Can you work these out from the model? Positions are in its coordinate system, mm. Face numbers are marked on the shaded views. A direction names the side the tool comes from. Give positions to 0.01 mm unless a question says otherwise; leave off trailing zeros. Loops run counter-clockwise (first coordinate to the right, second up) from the corner with the lowest first, then second, coordinate; pieces in that order, holes last. Notation, with made-up numbers: M -7,13.25 L 38,13.25 A32 cw 38,47.25 Z; hole C 73.5,75 d4. An arc over 180 degrees is marked long. Use CSV: the item, a comma, the result in double quotes.
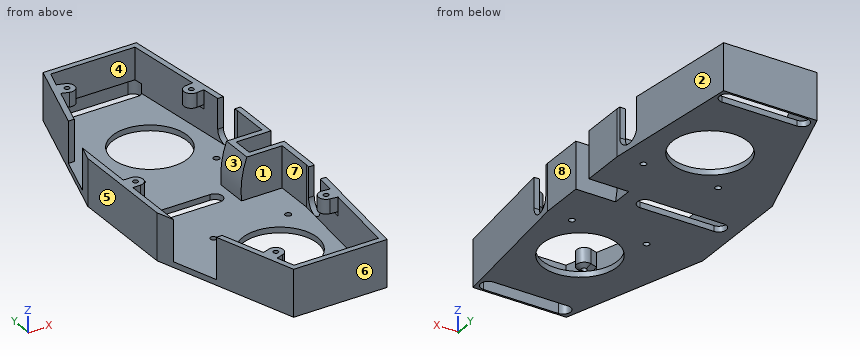
from build123d import *

# Parameters (mm, degrees)
EXTRUDE1_DEPTH          = 40
CHAMFER1_SIZE           = 20
CHAMFER1_SIZE2          = 11.547005384
CUT_EXTRUDE1_DEPTH      = 3
CUT_EXTRUDE1_DEPTH_BACK = 8
SKETCH4_R               = 45
SHELL2_T                = -3
SKETCH6_W               = 125.382075166
SKETCH6_H               = 262.961923039
CUT_EXTRUDE3_DEPTH      = 15
SKETCH7_W               = 55
SKETCH7_H               = 124
CUT_EXTRUDE4_DEPTH      = 22
CUT_EXTRUDE5_DEPTH      = 5
CUT_EXTRUDE5_DEPTH_BACK = 12
SKETCH8_R               = 20
SKETCH8_R_2             = 1.6
CUT_EXTRUDE6_DEPTH      = 10
SKETCH10_R              = 1.35
EXTRUDE2_DEPTH          = 10
CHAMFER2_SIZE           = 2.309401077
CHAMFER2_SIZE_2         = 4


with BuildPart() as part:
    # Sketch2 → Extrude1 (new body)
    with BuildSketch(Plane.XY):
        Polygon((24.967783135, -105), (33.5, -29), (33.5, 29), (24.967783135, 105), (-24.967783135, 105), (-49.5, 29), (-49.5, -29), (-24.967783135, -105), align=None)
    extrude(amount=EXTRUDE1_DEPTH)

    # Chamfer1
    chamfer1_edges = [part.edges().sort_by_distance(p)[0] for p in [
        (0, -105, 40),
        (29.233891568, -67, 40),
        (33.5, 0, 40),
        (29.233891568, 67, 40),
        (0, 105, 40),
        (-37.233891568, 67, 40),
        (-49.5, 0, 40),
        (-37.233891568, -67, 40),
    ]]
    chamfer1_side = [part.faces().sort_by_distance(p)[0] for p in [
        (-5.515477183, 0, 40),
    ]]
    chamfer(chamfer1_edges, length=CHAMFER1_SIZE, length2=CHAMFER1_SIZE2, reference=chamfer1_side[0])

    # Sketch4 → Cut-Extrude1 (cut, two sides: drawn at the far end of the back side and taken through both)
    with BuildSketch(Plane.XZ.offset(2.5).offset(-CUT_EXTRUDE1_DEPTH_BACK)):
        with Locations((56.5, 8)):
            Circle(SKETCH4_R)
    extrude(amount=CUT_EXTRUDE1_DEPTH + CUT_EXTRUDE1_DEPTH_BACK, mode=Mode.SUBTRACT)

    # Shell2
    shell2_openings = [part.faces().sort_by_distance(p)[0] for p in [
        (-6.280046319, 0, 40),
    ]]
    offset(amount=SHELL2_T, openings=shell2_openings, kind=Kind.INTERSECTION)

    # Sketch6 → Cut-Extrude3 (cut)
    with BuildSketch(Plane.XY.offset(40)):
        with Locations((5.510547988, -25.491958467)):
            Rectangle(SKETCH6_W, SKETCH6_H)
    extrude(amount=-CUT_EXTRUDE3_DEPTH, mode=Mode.SUBTRACT)

    # Sketch7 → Cut-Extrude4 (cut)
    with BuildSketch(Plane.XY.offset(25)):
        with Locations((-19, 0)):
            Rectangle(SKETCH7_W, SKETCH7_H)
    extrude(amount=-CUT_EXTRUDE4_DEPTH, mode=Mode.SUBTRACT)

    # Sketch8 → Cut-Extrude5 (cut, two sides: drawn at the far end of the back side and taken through both)
    with BuildSketch(Plane.XY.offset(3).offset(-CUT_EXTRUDE5_DEPTH_BACK)):
        with Locations((0, 54.5)):
            Circle(SKETCH8_R)
        with Locations((0, -54.5)):
            Circle(SKETCH8_R)
        with Locations((19.967783135, -30)):
            Circle(SKETCH8_R_2)
        with Locations((-19.967783135, -30)):
            Circle(SKETCH8_R_2)
        with Locations((19.967783135, 30)):
            Circle(SKETCH8_R_2)
        with Locations((-19.967783135, 30)):
            Circle(SKETCH8_R_2)
        with BuildLine():
            Line((-20.032216865, 104), (19.967783135, 104))
            ThreePointArc((19.967783135, 104), (23.967783135, 100), (19.967783135, 96))
            Line((19.967783135, 96), (-20.032216865, 96))
            ThreePointArc((-20.032216865, 96), (-24.032216865, 100), (-20.032216865, 104))
        make_face()
        with BuildLine():
            Line((-20.032216865, -96), (19.967783135, -96))
            ThreePointArc((19.967783135, -96), (23.967783135, -100), (19.967783135, -104))
            Line((19.967783135, -104), (-20.032216865, -104))
            ThreePointArc((-20.032216865, -104), (-24.032216865, -100), (-20.032216865, -96))
        make_face()
        with BuildLine():
            Line((-39.5, 4), (0, 4))
            ThreePointArc((0, 4), (4, 0), (0, -4))
            Line((0, -4), (-39.5, -4))
            ThreePointArc((-39.5, -4), (-43.5, 0), (-39.5, 4))
        make_face()
    extrude(amount=CUT_EXTRUDE5_DEPTH + CUT_EXTRUDE5_DEPTH_BACK, mode=Mode.SUBTRACT)

    # Sketch9 → Cut-Extrude6 (cut)
    with BuildSketch(Plane(origin=(33.5, 0, 0), x_dir=(0, 0, -1), z_dir=(1, 0, 0))):
        with BuildLine():
            Line((-25, 43), (-9, 43))
            ThreePointArc((-9, 43), (-3, 37), (-9, 31))
            Line((-9, 31), (-25, 31))
            ThreePointArc((-25, 31), (-31, 37), (-25, 43))
        make_face()
        with BuildLine():
            Line((-25, -31), (-9, -31))
            ThreePointArc((-9, -31), (-3, -37), (-9, -43))
            Line((-9, -43), (-25, -43))
            ThreePointArc((-25, -43), (-31, -37), (-25, -31))
        make_face()
    extrude(amount=-CUT_EXTRUDE6_DEPTH, mode=Mode.SUBTRACT)

    # Sketch10 → Extrude2 (add)
    # profile 1 of 5: a face of its own
    with BuildSketch(Plane.XY.offset(25)):
        with BuildLine():
            Line((-25.855592129, 92.48350258), (-28.313074008, 84.870304644))
            Line((-28.313074008, 84.870304644), (-24.50647504, 83.641563704))
            ThreePointArc((-24.50647504, 83.641563704), (-19.471135132, 86.219421733), (-22.048993161, 91.25476164))
            Line((-22.048993161, 91.25476164), (-25.855592129, 92.48350258))
        make_face()
        with Locations((-23.2777341, 87.448162672)):
            Circle(SKETCH10_R, mode=Mode.SUBTRACT)
    # profile 2 of 5: a face of its own
    with BuildSketch(Plane.XY.offset(25)):
        with BuildLine():
            Line((-46.5, 4), (-46.5, -4))
            Line((-46.5, -4), (-42.5, -4))
            ThreePointArc((-42.5, -4), (-38.5, 0), (-42.5, 4))
            Line((-42.5, 4), (-46.5, 4))
        make_face()
        with Locations((-42.5, 0)):
            Circle(SKETCH10_R, mode=Mode.SUBTRACT)
    # profile 3 of 5: a face of its own
    with BuildSketch(Plane.XY.offset(25)):
        with BuildLine():
            Line((27.793778068, -52.937571221), (23.81874958, -52.491310627))
            ThreePointArc((23.81874958, -52.491310627), (19.397460498, -56.020078522), (22.926228393, -60.441367604))
            Line((22.926228393, -60.441367604), (26.901256881, -60.887628197))
            Line((26.901256881, -60.887628197), (27.793778068, -52.937571221))
        make_face()
        with Locations(Location((23.372488986, -56.466339116, 0), (0, 0, 180))):
            Circle(SKETCH10_R, mode=Mode.SUBTRACT)
    # profile 4 of 5: a face of its own
    with BuildSketch(Plane.XY.offset(25)):
        with BuildLine():
            Line((26.901256881, 60.887628197), (27.793778068, 52.937571221))
            Line((27.793778068, 52.937571221), (23.81874958, 52.491310627))
            ThreePointArc((23.81874958, 52.491310627), (19.397460498, 56.020078522), (22.926228393, 60.441367604))
            Line((22.926228393, 60.441367604), (26.901256881, 60.887628197))
        make_face()
        with Locations((23.372488986, 56.466339116)):
            Circle(SKETCH10_R, mode=Mode.SUBTRACT)
    # profile 5 of 5: a face of its own
    with BuildSketch(Plane.XY.offset(25)):
        with BuildLine():
            Line((-28.313074008, -84.870304644), (-24.50647504, -83.641563704))
            ThreePointArc((-24.50647504, -83.641563704), (-19.471135132, -86.219421733), (-22.048993161, -91.25476164))
            Line((-22.048993161, -91.25476164), (-25.855592129, -92.48350258))
            Line((-25.855592129, -92.48350258), (-28.313074008, -84.870304644))
        make_face()
        with Locations(Location((-23.2777341, -87.448162672, 0), (0, 0, 180))):
            Circle(SKETCH10_R, mode=Mode.SUBTRACT)
    extrude(amount=-EXTRUDE2_DEPTH)

    # Chamfer2
    # the kernel refuses this chamfer: 4, 2.309401077 mm, written as the material it takes off along each edge
    with BuildSketch(Plane(origin=(22.926228393, 60.441367604, 15), x_dir=(0, 0, 1), z_dir=(0.9937571220719369, 0.11156514837215789, 0)), Plane(origin=(-22.048993161, -91.25476164, 15), x_dir=(0, 0, 1), z_dir=(-0.9516497420147145, -0.30718523487193755, 0))) as chamfer2_piece_1:
        Polygon((CHAMFER2_SIZE, 0), (0, CHAMFER2_SIZE_2), (0, 0), align=None)
    extrude(amount=4, mode=Mode.SUBTRACT)
    with BuildSketch(Plane(origin=(23.372488986, 56.466339116, 15), x_dir=(0.11156514837215781, -0.993757122071937, 0), z_dir=(0.993757122071937, 0.11156514837215781, 0))) as chamfer2_piece_2:
        Polygon((4 - CHAMFER2_SIZE_2, 0), (4, -CHAMFER2_SIZE), (4, 0), align=None)
    revolve(axis=Axis((23.372488986, 56.466339116, 15), (0, 0, -1)), revolution_arc=180, mode=Mode.SUBTRACT)
    with BuildSketch(Plane(origin=(27.793778068, 52.937571221, 15), x_dir=(-0.11156514837215799, 0.993757122071937, 0), z_dir=(-0.9937571220719369, -0.11156514837215799, 0)), Plane(origin=(-28.313074008, -84.870304644, 15), x_dir=(0.3071852348719375, -0.9516497420147145, 0), z_dir=(0.9516497420147145, 0.30718523487193755, 0))) as chamfer2_piece_3:
        Polygon((CHAMFER2_SIZE_2, 0), (0, -CHAMFER2_SIZE), (0, 0), align=None)
    extrude(amount=4, mode=Mode.SUBTRACT)
    with BuildSketch(Plane(origin=(-42.5, 4, 15), x_dir=(0, -1, 0), z_dir=(-1, 0, 0)), Plane(origin=(-22.048993161, 91.25476164, 15), x_dir=(-0.3071852348719375, -0.9516497420147145, 0), z_dir=(-0.9516497420147145, 0.30718523487193755, 0)), Plane(origin=(22.926228393, -60.441367604, 15), x_dir=(0.11156514837215789, 0.993757122071937, 0), z_dir=(0.9937571220719369, -0.11156514837215789, 0))) as chamfer2_piece_4:
        Polygon((CHAMFER2_SIZE_2, 0), (0, CHAMFER2_SIZE), (0, 0), align=None)
    extrude(amount=4, mode=Mode.SUBTRACT)
    with BuildSketch(Plane(origin=(-42.5, 0, 15), x_dir=(0, -1, 0), z_dir=(-1, 0, 0))) as chamfer2_piece_5:
        Polygon((4 - CHAMFER2_SIZE_2, 0), (4, CHAMFER2_SIZE), (4, 0), align=None)
    revolve(axis=Axis((-42.5, 0, 15), (0, 0, 1)), revolution_arc=180, mode=Mode.SUBTRACT)
    with BuildSketch(Plane(origin=(-46.5, -4, 15), x_dir=(0, 0, 1), z_dir=(1, 0, 0)), Plane(origin=(-28.313074008, 84.870304644, 15), x_dir=(0, 0, 1), z_dir=(0.9516497420147144, -0.30718523487193783, 0)), Plane(origin=(27.793778068, -52.937571221, 15), x_dir=(0, 0, 1), z_dir=(-0.9937571220719369, 0.11156514837215789, 0))) as chamfer2_piece_6:
        Polygon((CHAMFER2_SIZE, 0), (0, -CHAMFER2_SIZE_2), (0, 0), align=None)
    extrude(amount=4, mode=Mode.SUBTRACT)
    with BuildSketch(Plane(origin=(-23.2777341, 87.448162672, 15), x_dir=(-0.3071852348719437, -0.9516497420147125, 0), z_dir=(-0.9516497420147125, 0.3071852348719437, 0))) as chamfer2_piece_7:
        Polygon((4 - CHAMFER2_SIZE_2, 0), (4, CHAMFER2_SIZE), (4, 0), align=None)
    revolve(axis=Axis((-23.2777341, 87.448162672, 15), (0, 0, 1)), revolution_arc=180, mode=Mode.SUBTRACT)
    with BuildSketch(Plane(origin=(-23.2777341, -87.448162672, 15), x_dir=(-0.3071852348719429, 0.9516497420147128, 0), z_dir=(-0.9516497420147128, -0.3071852348719429, 0))) as chamfer2_piece_8:
        Polygon((4 - CHAMFER2_SIZE_2, 0), (4, -CHAMFER2_SIZE), (4, 0), align=None)
    revolve(axis=Axis((-23.2777341, -87.448162672, 15), (0, 0, -1)), revolution_arc=180, mode=Mode.SUBTRACT)
    with BuildSketch(Plane(origin=(23.372488986, -56.466339116, 15), x_dir=(0.11156514837215692, 0.993757122071937, 0), z_dir=(0.993757122071937, -0.11156514837215692, 0))) as chamfer2_piece_9:
        Polygon((4 - CHAMFER2_SIZE_2, 0), (4, CHAMFER2_SIZE), (4, 0), align=None)
    revolve(axis=Axis((23.372488986, -56.466339116, 15), (0, 0, 1)), revolution_arc=180, mode=Mode.SUBTRACT)


solid = part.part
Q1. I want a section at C-C, the plane y = -26. Please give me the cut outline in (x, z).
Model answer:
outline,"M -49.5,0 L 33.5,0 L 33.5,25 L 30.5,25 L 30.5,3 L -46.5,3 L -46.5,25 L -49.5,25 Z"
Q2. For the marked faces 1, 2, 3, 4 and 5, which set-ups out of +Z, -Z, +X, -X, +Y, -Y let a thin tool reach every point of the face, with its end or its side?
Model answer:
face 1,"+Z"
face 2,"+Z, -Z, +X, +Y"
face 3,"none"
face 4,"+Z, -Z"
face 5,"+Z, -Z, -X, +Y, -Y"
Q3. Please list where these lines run through material, in increasing order: L1, parallel to Y at x = 11, z = 6.5; L2, parallel to Y at x = 20.5, z = 14.5; L3, parallel to Y at x = -42.5, z = 22.75. Write a range as from..to.
Model answer:
L1,"-105..-104, -8.5..8.5, 104..105"
L2,"-105..-102, -8.5..-5.5, 5.5..8.5, 102..105"
L3,"-4..-1.35, 1.35..4"
Q4. If we mould it in two halves opening along Y, with no side actions, what happens to the marked faces 6, 7 and 8? For each: released by +Y, released by -Y, zero draft, split by the parting line, or undercut.
Model answer:
face 6,"released by -Y"
face 7,"undercut"
face 8,"zero draft"
Q5. I'm going to push flat-ended pins straight in: P1, Ø8, axis at y = 63, z = 22.5, coming from the -X side; P2, Ø2, axis at x = -1, y = -81.5, coming from the +Z side; P3, Ø3.5, axis at x = -0.5, y = 99.5, coming from the -Z side; P4, Ø2, axis at x = -44, z = 20, coming from the -Y side. Where does each tip first touch, or does it pass through?
Model answer:
P1,"x = -38.85"
P2,"z = 3"
P3,"through"
P4,"y = -4"
Q6. I want a section at A-A, the plane y = -64. Please give me the cut outline in (x, z), then the cut area to 3 significant figures.
Model answer:
outline,"M -38.2,0 L -17.6,0 L -17.6,3 L -35.05,3 L -35.05,25 L -38.2,25 Z; M 17.6,0 L 29.57,0 L 29.57,25 L 26.55,25 L 26.55,3 L 17.6,3 Z"
area,"233 mm2"
Q7. I want a section at B-B, the plane z = 22. State how many separate pieces and enclosed holes the cut face has, then the cut area to 3 significant figures.
Model answer:
separate pieces,"4"
enclosed holes,"5"
area,"1,680 mm2"
